Check sheet for the modelled part. Datum: model origin and axes. Units: mm. A direction names the side the tool comes from. Give positions to 0.01 mm unless a question says otherwise; leave off trailing zeros. Loops run counter-clockwise (first coordinate to the right, second up) from the corner with the lowest first, then second, coordinate; pieces in that order, holes last. Notation, with made-up numbers: (42.25, 52) -> (55.25, 52) arc R22 ccw to (55.25, 82) -> close; hole circle Ø9 at (17.25, -10.5). An arc over 180 degrees is marked (long way). Write each question's results on one line, items separated by ' | '. Start each with the question number.
1. Cross-section at A-A on x = -9.5. Record the boundary of the cut face in (y, z).
2. Cross-section at D-D on x = -25.5. Record the boundary of the cut face in (y, z), and give its area (3 significant figures).
3. Cross-section at C-C on y = 9. Record the boundary of the cut face in (x, z), and give its area (3 significant figures).
4. Cross-section at B-B on z = 0. Record the boundary of the cut face in (x, y).
5. Gauge pin test, flat ends, axial feed: pin 1 Ø11 at (x, y) = (-10.5, 15.5) entering from -Z; pin 2 Ø3 at (x, z) = (-20, -16.5) entering from -Y; pin 3 Ø15 at (x, z) = (-18, -23) entering from +Y; pin 4 Ø1.4 at (y, z) = (3.5, -23) entering from +X. Record the tip position at first contact, or that the pin passes through.
6. Material ranges on L1, parallel to Z at x = -29, y = 12.5; L2, parallel to Y at x = -1.5, z = -5; L3, parallel to Y at x = -18.5, z = 6, recorded low to high. Write a range as from..to.
7. Tool access check on faces 1 (the face through (-12.81, 32.37, 5.05)), 2 (the face through (-15, 4.542, -24)), 3 (the face through (-22.121, 2, -24)), 4 (the face through (-15, 0, 3)), 5 (the face through (-8.268, 2, -24)). Record the directions out of +Z, -Z, +X, -X, +Y, -Y that give a thin tool (end or side, any length) a straight path to the whole face; none if there is none.
from build123d import *

# Parameters (mm, degrees)
SKETCH1_W           = 42.3
SKETCH1_H           = 42.3
BOSS_EXTRUDE1_DEPTH = 21.5
SKETCH2_R           = 11
BOSS_EXTRUDE2_DEPTH = 2
SKETCH3_R           = 2.5
BOSS_EXTRUDE3_DEPTH = 18
SKETCH4_W           = 13.852605362
SKETCH4_H           = 4.542451726
BOSS_EXTRUDE4_DEPTH = 17


with BuildPart() as part:
    # Sketch1 → Boss-Extrude1 (new body)
    with BuildSketch(Plane(origin=(0, 0, 0), x_dir=(1, 0, 0), z_dir=(0, 1, 0))):
        with Locations((-15.194404332, -5.802888087)):
            Rectangle(SKETCH1_W, SKETCH1_H)
    extrude(amount=BOSS_EXTRUDE1_DEPTH)

    # Sketch2 → Boss-Extrude2 (add)
    with BuildSketch(Plane(origin=(0, 21.5, 0), x_dir=(1, 0, 0), z_dir=(0, 1, 0))):
        with Locations((-15.194404332, -5.802888087)):
            Circle(SKETCH2_R)
    extrude(amount=BOSS_EXTRUDE2_DEPTH)

    # Sketch3 → Boss-Extrude3 (add)
    with BuildSketch(Plane(origin=(0, 23.5, 0), x_dir=(1, 0, 0), z_dir=(0, 1, 0))):
        with Locations((-15.194404332, -5.802888087)):
            Circle(SKETCH3_R)
    extrude(amount=BOSS_EXTRUDE3_DEPTH)

    # Sketch4 → Boss-Extrude4 (add)
    with BuildSketch(Plane(origin=(0, 0, -15.347111913), x_dir=(-1, 0, 0), z_dir=(0, 0, -1))):
        with Locations((15.194404332, 2.271225863)):
            Rectangle(SKETCH4_W, SKETCH4_H)
    extrude(amount=BOSS_EXTRUDE4_DEPTH)


solid = part.part
Geometry says:
1) outline: (0, -32.35) -> (4.54, -32.35) -> (4.54, -15.35) -> (21.5, -15.35) -> (21.5, -3.61) -> (23.5, -3.61) -> (23.5, 15.21) -> (21.5, 15.21) -> (21.5, 26.95) -> (0, 26.95) -> close
2) outline: (0, -15.35) -> (21.5, -15.35) -> (21.5, 1.96) -> (23.5, 1.96) -> (23.5, 9.65) -> (21.5, 9.65) -> (21.5, 26.95) -> (0, 26.95) -> close | area: 925 mm^2
3) outline: (-36.34, -15.35) -> (5.96, -15.35) -> (5.96, 26.95) -> (-36.34, 26.95) -> close | area: 1,790 mm^2
4) outline: (-36.34, 0) -> (5.96, 0) -> (5.96, 21.5) -> (-5.85, 21.5) -> (-5.85, 23.5) -> (-24.54, 23.5) -> (-24.54, 21.5) -> (-36.34, 21.5) -> close
5) pin 1: z = -15.35 | pin 2: y = 0 | pin 3: y = 4.54 | pin 4: x = -8.27
6) L1: -15.35..26.95 | L2: 0..21.5 | L3: 0..23.5
7) face 1: +Y | face 2: -Z, +X, -X, +Y | face 3: -Z, -X, +Y, -Y | face 4: +Z, -Z, +X, -X, -Y | face 5: -Z, +X, +Y, -Y
